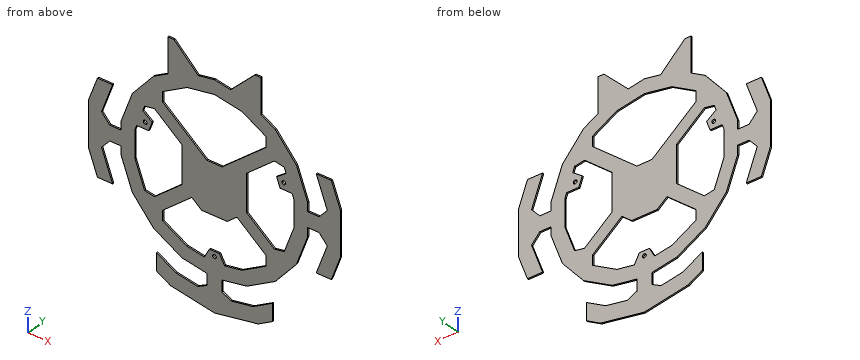
```python
from build123d import *

# Parameters (mm, degrees)
BOSS_EXTRUDE1_DEPTH    = 1.2
BOSS_EXTRUDE17_DEPTH   = 1.2
BOSS_EXTRUDE17_2_DEPTH = 1.2
BOSS_EXTRUDE17_3_DEPTH = 1.2
SKETCH18_W             = 18
SKETCH18_H             = 12
BOSS_EXTRUDE18_DEPTH   = 1.2
BOSS_EXTRUDE19_DEPTH   = 1.2
BOSS_EXTRUDE20_DEPTH   = 1.2
BOSS_EXTRUDE21_DEPTH   = 1.2
BOSS_EXTRUDE22_DEPTH   = 1.2
BOSS_EXTRUDE23_DEPTH   = 1.2
BOSS_EXTRUDE26_DEPTH   = 1.2
BOSS_EXTRUDE29_DEPTH   = 1.2
BOSS_EXTRUDE30_DEPTH   = 1.2
BOSS_EXTRUDE31_DEPTH   = 1.2
SKETCH37_R             = 1.5
CUT_EXTRUDE1_DEPTH     = 1.2
SKETCH38_R             = 1.5
CUT_EXTRUDE2_DEPTH     = 1.2
BOSS_EXTRUDE32_DEPTH   = 1.2


with BuildPart() as part:
    # Sketch1 → Boss-Extrude1 (new body)
    with BuildSketch(Plane(origin=(0, 0, 0), x_dir=(1, 0, 0), z_dir=(0, 1, 0))):
        Polygon((0, 75), (-25.651510749, 70.476946559), (-48.209070726, 57.453333234), (-64.951905284, 37.5), (-73.860581476, 13.023613325), (-73.860581476, -13.023613325), (-64.951905284, -37.5), (-48.209070726, -57.453333234), (-25.651510749, -70.476946559), (0, -75), (25.651510749, -70.476946559), (48.209070726, -57.453333234), (64.951905284, -37.5), (73.860581476, -13.023613325), (73.860581476, 13.023613325), (64.951905284, 37.5), (48.209070726, 57.453333234), (25.651510749, 70.476946559), align=None)
        Polygon((0, 63.830307269), (-21.831250841, 59.980868723), (-41.029330635, 48.896852186), (-55.278667627, 31.915153635), (-62.860581476, 11.084016537), (-62.860581476, -11.084016537), (-55.278667627, -31.915153635), (-41.029330635, -48.896852186), (-21.831250841, -59.980868723), (0, -63.830307269), (21.831250841, -59.980868723), (41.029330635, -48.896852186), (55.278667627, -31.915153635), (62.860581476, -11.084016537), (62.860581476, 11.084016537), (55.278667627, 31.915153635), (41.029330635, 48.896852186), (21.831250841, 59.980868723), align=None, mode=Mode.SUBTRACT)
    extrude(amount=BOSS_EXTRUDE1_DEPTH)



with BuildPart() as body_2:
    # Sketch15 → Boss-Extrude17 (new body)
    with BuildSketch(Plane.XZ):
        Polygon((0, -101.401091909), (34.681215988, -95.285857807), (36.930290738, -93.987353894), (36.930290738, -84.749749587), (31.902845145, -87.652346653), (0, -93.277679014), (-31.902845145, -87.652346653), (-36.930290738, -84.749749587), (-36.930290738, -93.987353894), (-34.681215988, -95.285857807), align=None)
    extrude(amount=-BOSS_EXTRUDE17_DEPTH)


with BuildPart() as body_3:
    # Sketch15 → Boss-Extrude17 2 (new body)
    with BuildSketch(Plane.XZ):
        Polygon((92.620527368, -37.5), (99.860581476, -17.608114823), (99.860581476, 17.608114823), (92.620527368, 37.5), (84.107105188, 37.5), (91.860581476, 16.197498978), (91.860581476, -16.197498978), (84.107105188, -37.5), align=None)
    extrude(amount=-BOSS_EXTRUDE17_2_DEPTH)


with BuildPart() as body_4:
    # Sketch15 → Boss-Extrude17 3 (new body)
    with BuildSketch(Plane.XZ):
        Polygon((-92.620527368, 37.5), (-99.860581476, 17.608114823), (-99.860581476, -17.608114823), (-92.620527368, -37.5), (-84.107105188, -37.5), (-91.860581476, -16.197498978), (-91.860581476, 16.197498978), (-84.107105188, 37.5), align=None)
    extrude(amount=-BOSS_EXTRUDE17_3_DEPTH)


with BuildPart() as part_1:
    add(part.part)

    add(body_2.part)  # Boss-Extrude18 merges body 2

    add(body_3.part)  # Boss-Extrude18 merges body 3

    add(body_4.part)  # Boss-Extrude18 merges body 4
    # Sketch18 → Boss-Extrude18 (add)
    with BuildSketch(Plane.XZ):
        with Locations((-82.860581476, 0)):
            Rectangle(SKETCH18_W, SKETCH18_H)
        with Locations((82.860581476, 0)):
            Rectangle(SKETCH18_W, SKETCH18_H)
        Polygon((-6, -73.942038116), (-6, -92.21971713), (0, -93.277679014), (6, -92.21971713), (6, -73.942038116), (0, -75), align=None)
    extrude(amount=-BOSS_EXTRUDE18_DEPTH)

    # Sketch19 → Boss-Extrude19 (add)
    with BuildSketch(Plane.XZ):
        Polygon((-91.860581476, 16.197498978), (-82.860581476, 6), (-91.860581476, 6), align=None)
        Polygon((-91.860581476, -16.197498978), (-82.860581476, -6), (-91.860581476, -6), align=None)
        Polygon((91.860581476, 16.197498978), (82.860581476, 6), (91.860581476, 6), align=None)
        Polygon((91.860581476, -16.197498978), (82.860581476, -6), (91.860581476, -6), align=None)
        Polygon((18.951422573, -89.936031892), (6, -83.080877623), (6, -92.21971713), align=None)
        Polygon((-6, -83.080877623), (-6, -92.21971713), (-18.951422573, -89.936031892), align=None)
    extrude(amount=-BOSS_EXTRUDE19_DEPTH)

    # Sketch20 → Boss-Extrude20 (add)
    with BuildSketch(Plane.XZ):
        Polygon((-36.930290738, 63.965139896), (-36.930290738, 91.965139896), (-32.052421992, 91.965139896), (-12.825755375, 72.738473279), (-25.651510749, 70.476946559), align=None)
        Polygon((36.930290738, 63.965139896), (36.930290738, 91.965139896), (32.052421992, 91.965139896), (12.825755375, 72.738473279), (25.651510749, 70.476946559), align=None)
    extrude(amount=-BOSS_EXTRUDE20_DEPTH)

    # Sketch23 → Boss-Extrude21 (add)
    with BuildSketch(Plane(origin=(0, 1.2, 0), x_dir=(1, 0, 0), z_dir=(0, 1, 0))):
        Polygon((-92.620527368, 37.5), (-80.620527368, 37.5), (-89.392030332, 13.400493671), (-89.392030332, -13.400493671), (-80.620527368, -37.5), (-92.620527368, -37.5), (-99.860581476, -17.608114823), (-99.860581476, 17.608114823), align=None)
        Polygon((80.620527368, -37.5), (89.392030332, -13.400493671), (89.392030332, 13.400493671), (80.620527368, 37.5), (92.620527368, 37.5), (99.860581476, 17.608114823), (99.860581476, -17.608114823), (92.620527368, -37.5), align=None)
    extrude(amount=-BOSS_EXTRUDE21_DEPTH)

    # Sketch24 → Boss-Extrude22 (add)
    with BuildSketch(Plane(origin=(0, 1.2, 0), x_dir=(1, 0, 0), z_dir=(0, 1, 0))):
        Polygon((-36.930290738, 93.987353894), (-36.930290738, 80.130947434), (-30.513659724, 83.835591077), (-13.195234763, 86.889296661), (13.195234763, 86.889296661), (30.513659724, 83.835591077), (36.930290738, 80.130947434), (36.930290738, 93.987353894), (34.681215988, 95.285857807), (0, 101.401091909), (-34.681215988, 95.285857807), align=None)
    extrude(amount=-BOSS_EXTRUDE22_DEPTH)

    # Sketch26 → Boss-Extrude23 (add)
    with BuildSketch(Plane(origin=(0, 1.2, 0), x_dir=(1, 0, 0), z_dir=(0, 1, 0))):
        Polygon((-36.930290738, 93.987353894), (-45.930290738, 88.791201472), (-45.930290738, 74.934795011), (-36.930290738, 80.130947434), align=None)
        Polygon((36.930290738, 93.987353894), (45.930290738, 88.791201472), (45.930290738, 74.934795011), (36.930290738, 80.130947434), align=None)
    extrude(amount=-BOSS_EXTRUDE23_DEPTH)

    # Sketch27 → Boss-Extrude26 (add)
    with BuildSketch(Plane.XZ):
        Polygon((-44.940061082, 44.236225126), (0, 6.527036447), (44.940061082, 44.236225126), (51.367937179, 36.575780695), (7.778619134, 0), (51.367937179, -36.575780695), (44.940061082, -44.236225126), (0, -6.527036447), (-44.940061082, -44.236225126), (-51.367937179, -36.575780695), (-7.778619134, 0), (-51.367937179, 36.575780695), align=None)
    extrude(amount=-BOSS_EXTRUDE26_DEPTH)

    # Sketch31 → Boss-Extrude29 (add)
    with BuildSketch(Plane.XZ):
        Polygon((-10.098423643, -28), (10.098423643, -28), (25.590481458, -15.054072893), (25.590481458, 14.945927107), (6, 11.561634234), (-6, 11.561634234), (-25.590481458, 14.945927107), (-25.590481458, -15.054072893), align=None)
    extrude(amount=-BOSS_EXTRUDE29_DEPTH)

    # Sketch32 → Boss-Extrude30 (add)
    with BuildSketch(Plane(origin=(0, 1.2, 0), x_dir=(1, 0, 0), z_dir=(0, 1, 0))):
        Polygon((-41.029330635, 48.896852186), (-41.029330635, 40.95473265), (-44.940061082, 44.236225126), align=None)
        Polygon((41.029330635, 48.896852186), (41.029330635, 40.95473265), (44.940061082, 44.236225126), align=None)
        Polygon((44.940061082, -44.236225126), (41.029330635, -48.896852186), (41.029330635, -40.95473265), align=None)
        Polygon((-41.029330635, -48.896852186), (-41.029330635, -40.95473265), (-44.940061082, -44.236225126), align=None)
    extrude(amount=-BOSS_EXTRUDE30_DEPTH)

    # Sketch34 → Boss-Extrude31 (add)
    with BuildSketch(Plane(origin=(0, 1.2, 0), x_dir=(1, 0, 0), z_dir=(0, 1, 0))):
        Polygon((8, 62.419691424), (4, 54.830307269), (-4, 54.830307269), (-8, 62.419691424), (0, 63.830307269), align=None)
        Polygon((-61.55807149, -14.662633313), (-56.769789483, -27.818330004), (-49.244310391, -22.180174279), (-50.612390964, -18.421403796), (-51.980471537, -14.662633313), align=None)
        Polygon((50.612390964, -18.421403796), (49.244310391, -22.180174279), (56.769789483, -27.818330004), (61.55807149, -14.662633313), (51.980471537, -14.662633313), align=None)
    extrude(amount=-BOSS_EXTRUDE31_DEPTH)

    # Sketch37 → Cut-Extrude1 (cut)
    with BuildSketch(Plane(origin=(0, 1.2, 0), x_dir=(1, 0, 0), z_dir=(0, 1, 0))):
        with Locations(Location((-54.84814578, -19.96309247, 0), (0, 0, 270))):
            Circle(SKETCH37_R)
        with Locations(Location((54.84814578, -19.96309247, 0), (0, 0, 270))):
            Circle(SKETCH37_R)
    extrude(amount=-CUT_EXTRUDE1_DEPTH, mode=Mode.SUBTRACT)

    # Sketch38 → Cut-Extrude2 (cut)
    with BuildSketch(Plane(origin=(0, 1.2, 0), x_dir=(1, 0, 0), z_dir=(0, 1, 0))):
        with Locations(Location((0, 58.81204127, 0), (0, 0, 270))):
            Circle(SKETCH38_R)
    extrude(amount=-CUT_EXTRUDE2_DEPTH, mode=Mode.SUBTRACT)

    # Sketch39 → Boss-Extrude32 (add)
    with BuildSketch(Plane(origin=(0, 1.2, 0), x_dir=(1, 0, 0), z_dir=(0, 1, 0))):
        Polygon((-51.367937179, 36.575780695), (-47.457206732, 33.294288219), (-55.278667627, 31.915153635), align=None)
        Polygon((51.367937179, 36.575780695), (55.278667627, 31.915153635), (47.457206732, 33.294288219), align=None)
        Polygon((51.367937179, -36.575780695), (55.278667627, -31.915153635), (47.457206732, -33.294288219), align=None)
        Polygon((-47.457206732, -33.294288219), (-51.367937179, -36.575780695), (-55.278667627, -31.915153635), align=None)
    extrude(amount=-BOSS_EXTRUDE32_DEPTH)


solid = part_1.part
```
Verification items for the finished model (mm, model axes). Give positions to 0.01 mm unless a question says otherwise; leave off trailing zeros. Order: outer loops, then holes, each group sorted by start corner. A loop starts at its lowest first (then second) coordinate and runs counter-clockwise, first axis right, second up. Notation, with made-up numbers: M 79.5,-16.5 L 96.5,-16.5 A15 cw 96.5,-2.5 Z; hole C 54,62 d2. An arc over 180 degrees is marked long. Answer in a Markdown table with one row per item. Add a question column.
Item 1: Gauge pin test, flat end, axial feed: pin 1 (12 mm diameter, centred on x = 62.5, z = 58.5, fed in from +Y). Record the tip position at first contact, or that the pin passes through.
Item 2: Section check A-A, the plane z = -2. Enter the section's corners in (x, y), and give its area (3 significant figures).
Item 3: Section check C-C, the plane y = 0.8. State how many separate pieces and enclosed holes the cut face has, and give its area (3 significant figures).
Item 4: Section check B-B, the plane z = 55. Enter the section's corners in (x, y).
Item 5: Scan lines: probe 1 along X at (y, z) = (0.6, 1.5); probe 2 along Z at (x, y) = (-30.5, 0.45); probe 3 along Z at (x, y) = (-39, 0.7). Record each from-to range of solid material in increasing order. Write a range as from..to.
Item 6: Section check D-D, the plane x = -68.5. Enter the section's corners in (y, z), and give its area (3 significant figures).
Filled sheet:
| question | item | result |
|---|---|---|
| 1 | pin 1 | passes through |
| 2 | outline | M -99.86,0 L -62.86,0 L -62.86,1.2 L -99.86,1.2 Z; M -25.59,0 L 25.59,0 L 25.59,1.2 L -25.59,1.2 Z; M 62.86,0 L 99.86,0 L 99.86,1.2 L 62.86,1.2 Z |
| 2 | area | 150 mm^2 |
| 3 | separate pieces | 1 |
| 3 | enclosed holes | 7 |
| 3 | area | 12,900 mm^2 |
| 4 | outline | M -50.27,0 L -30.46,0 L -30.46,1.2 L -50.27,1.2 Z; M 30.46,0 L 50.27,0 L 50.27,1.2 L 30.46,1.2 Z |
| 5 | probe 1 | x = -99.86..-62.86, -25.59..25.59, 62.86..99.86 |
| 5 | probe 2 | z = -96.02..-83.84, -67.68..-54.98, -32.12..-19.07, 19.07..32.12, 54.98..90.41 |
| 5 | probe 3 | z = -92.79..-78.94, -62.77..-50.07, -39.25..-26.2, 26.2..39.25, 50.07..62.77 |
| 6 | outline | M 0,-27.75 L 1.2,-27.75 L 1.2,27.75 L 0,27.75 Z |
| 6 | area | 66.6 mm^2 |
